Source: CAD feature listing. Evaluate the final solid. Frame: model axes, mm. A direction names the side the tool comes from. Give positions to 0.01 mm unless a question says otherwise; leave off trailing zeros. Order: outer loops, then holes, each group sorted by start corner. A loop starts at its lowest first (then second) coordinate and runs counter-clockwise, first axis right, second up. Notation, with made-up numbers: M -28.75,20 L 20.25,20 A33 ccw 20.25,49 Z; hole C 42.25,88 d8. An arc over 180 degrees is marked long. Use CSV: the item, a comma, the result in double quotes. Start each with the question number.
1. Section query B-B, the plane y = 10.5. Return the cut outline in (x, z).
2. Section query C-C, the plane x = 8.5. Return the cut outline in (y, z), plus the area to 3 significant figures.
3. Pin query (flat end, axial travel): P1, Ø0.8, axis at y = 47.5, z = 21.5, coming from the -X side; P2, Ø1.1, axis at x = 27, z = 20.5, coming from the -Y side; P3, Ø1.7, axis at x = -30, z = -17.5, coming from the -Y side; P4, Ø3, axis at y = 47.5, z = 21, coming from the +X side. Return the tip coordinate at first contact, or that it passes through.
4. Mould query, pull axis X, two halves, no side actions, for faces 4 (the flat face through (30, 2, -13)), 5 (the flat face through (-35, 29, 0)), 6 (the flat face through (0, 29, -22.5)). Classes: released by +X, released by -X, zero draft, split by the parting line, or undercut.
5. Line query: line 1 along X through (y, z) = (9, -11.5); line 2 along X through (y, z) = (1, 17); line 3 along Z through (x, y) = (-1, 14). Output: solid intervals per line, ascending. Write a range as [from, to].
6. Reachability of faces 1 (the flat face through (32.591, 30, 0)), 2 (the flat face through (-26.25, 47, 21)), 3 (the flat face through (30, 2, 13)) from +Z, -Z, +X, -X, +Y, -Y: full face, straight path, thin tool, end or side. Return the list, or none.
7. Section query D-D, the plane z = 0. Return the cut outline in (x, y).
8. Section query A-A, the plane x = 1.5. Return the cut outline in (y, z).
from build123d import *

# Parameters (mm, degrees)
SKETCH_1_W          = 70
SKETCH_1_H          = 45
EXTRUDE_1_DEPTH     = 3
SKETCH_2_W          = 13
SKETCH_2_H          = 23
CUT_EXTRUDE_1_DEPTH = 10
SKETCH_3_R          = 0.95
CUT_EXTRUDE_2_DEPTH = 10
FILLET_1_R          = 5
FILLET_2_R          = 5
SKETCH_4_R          = 0.95
CUT_EXTRUDE_3_DEPTH = 10
CUT_EXTRUDE_4_DEPTH = 10
SKETCH_9_W          = 65.182596022
SKETCH_9_H          = 39.488918008
EXTRUDE_2_DEPTH     = 55
SKETCH_10_W         = 1
SKETCH_10_H         = 2.5
SKETCH_10_W_2       = 15
SKETCH_10_H_2       = 10
CUT_EXTRUDE_5_DEPTH = 7


with BuildPart() as part:
    # 草图1 → 凸台-拉伸1 (new body)
    with BuildSketch(Plane(origin=(0, 0, 0), x_dir=(1, 0, 0), z_dir=(0, 1, 0))):
        Rectangle(SKETCH_1_W, SKETCH_1_H)
    extrude(amount=EXTRUDE_1_DEPTH)

    # 草图2 → 切除-拉伸1 (cut)
    with BuildSketch(Plane(origin=(0, 3, 0), x_dir=(1, 0, 0), z_dir=(0, 1, 0))):
        with Locations((24, 0)):
            Rectangle(SKETCH_2_W, SKETCH_2_H)
        with Locations((-24, 0)):
            Rectangle(SKETCH_2_W, SKETCH_2_H)
    extrude(amount=-CUT_EXTRUDE_1_DEPTH, mode=Mode.SUBTRACT)

    # 草图3 → 切除-拉伸2 (cut)
    with BuildSketch(Plane(origin=(0, 3, 0), x_dir=(1, 0, 0), z_dir=(0, 1, 0))):
        with Locations((-24, 14)):
            Circle(SKETCH_3_R)
        with Locations((-24, -14)):
            Circle(SKETCH_3_R)
        with Locations((24, 14)):
            Circle(SKETCH_3_R)
        with Locations((24, -14)):
            Circle(SKETCH_3_R)
    extrude(amount=-CUT_EXTRUDE_2_DEPTH, mode=Mode.SUBTRACT)

    # 圆角1
    fillet_1_edges = [part.edges().sort_by_distance(p)[0] for p in [
        (35, 1.5, -22.5),
    ]]
    fillet(fillet_1_edges, radius=FILLET_1_R)

    # 圆角2
    fillet_2_edges = [part.edges().sort_by_distance(p)[0] for p in [
        (35, 1.5, 22.5),
        (-35, 1.5, 22.5),
        (-35, 1.5, -22.5),
    ]]
    fillet(fillet_2_edges, radius=FILLET_2_R)

    # 草图4 → 切除-拉伸3 (cut)
    with BuildSketch(Plane(origin=(0, 3, 0), x_dir=(1, 0, 0), z_dir=(0, 1, 0))):
        with Locations((-30, 17.5)):
            Circle(SKETCH_4_R)
        with Locations((30, 17.5)):
            Circle(SKETCH_4_R)
        with Locations((-30, -17.5)):
            Circle(SKETCH_4_R)
        with Locations((30, -17.5)):
            Circle(SKETCH_4_R)
    extrude(amount=-CUT_EXTRUDE_3_DEPTH, mode=Mode.SUBTRACT)

    # 草图8 → 切除-拉伸4 (cut)
    with BuildSketch(Plane(origin=(0, 3, 0), x_dir=(1, 0, 0), z_dir=(0, 1, 0))):
        with BuildLine():
            Line((-27, 17.5), (27, 17.5))
            ThreePointArc((27, 17.5), (27.878679656, 15.378679656), (30, 14.5))
            Line((30, 14.5), (30, -14.5))
            ThreePointArc((30, -14.5), (27.878679656, -15.378679656), (27, -17.5))
            Line((27, -17.5), (-27, -17.5))
            ThreePointArc((-27, -17.5), (-27.878679656, -15.378679656), (-30, -14.5))
            Line((-30, -14.5), (-30, 14.5))
            ThreePointArc((-30, 14.5), (-27.878679656, 15.378679656), (-27, 17.5))
        make_face()
    extrude(amount=-CUT_EXTRUDE_4_DEPTH, mode=Mode.SUBTRACT)

    # 草图9 → 凸台-拉伸2 (add)
    with BuildSketch(Plane(origin=(0, 3, 0), x_dir=(1, 0, 0), z_dir=(0, 1, 0))):
        with BuildLine():
            Line((-30, -22.5), (30, -22.5))
            ThreePointArc((30, -22.5), (33.535533906, -21.035533906), (35, -17.5))
            Line((35, -17.5), (35, 17.5))
            ThreePointArc((35, 17.5), (33.535533906, 21.035533906), (30, 22.5))
            Line((30, 22.5), (-30, 22.5))
            ThreePointArc((-30, 22.5), (-33.535533906, 21.035533906), (-35, 17.5))
            Line((-35, 17.5), (-35, -17.5))
            ThreePointArc((-35, -17.5), (-33.535533906, -21.035533906), (-30, -22.5))
        make_face()
        Rectangle(SKETCH_9_W, SKETCH_9_H, mode=Mode.SUBTRACT)
    extrude(amount=EXTRUDE_2_DEPTH)

    # 草图10 → 切除-拉伸5 (cut)
    with BuildSketch(Plane(origin=(0, 0, 22.5), x_dir=(-1, 0, 0), z_dir=(0, 0, -1))):
        with Locations((26.75, 6.25)):
            Rectangle(SKETCH_10_W, SKETCH_10_H)
        with Locations((26.75, 47.25)):
            Rectangle(SKETCH_10_W, SKETCH_10_H)
        with Locations((-26.75, 21.25)):
            Rectangle(SKETCH_10_W, SKETCH_10_H)
        with Locations((-26.75, 47.25)):
            Rectangle(SKETCH_10_W, SKETCH_10_H)
        with Locations((0, 43)):
            Rectangle(SKETCH_10_W_2, SKETCH_10_H_2)
    extrude(amount=CUT_EXTRUDE_5_DEPTH, mode=Mode.SUBTRACT)


solid = part.part
Result set:
1,outline,"M -35,-17.5 A5 ccw -30,-22.5 L 30,-22.5 A5 ccw 35,-17.5 L 35,17.5 A5 ccw 30,22.5 L -30,22.5 A5 ccw -35,17.5 Z; hole M -32.59,-19.74 L 32.59,-19.74 L 32.59,19.74 L -32.59,19.74 Z"
2,outline,"M 0,-22.5 L 58,-22.5 L 58,-19.74 L 3,-19.74 L 3,-17.5 L 0,-17.5 Z; M 0,17.5 L 3,17.5 L 3,19.74 L 58,19.74 L 58,22.5 L 0,22.5 Z"
2,area,"333 mm2"
3,P1,"x = -33.47"
3,P2,"y = 0"
3,P3,"through"
3,P4,"x = 34.58"
4,face 4,"undercut"
4,face 5,"released by -X"
4,face 6,"zero draft"
5,line 1,"[-35, -32.59], [32.59, 35]"
5,line 2,"[-35, -30.81], [-29.19, -27.04], [27.04, 29.19], [30.81, 35]"
5,line 3,"[-22.5, -19.74], [19.74, 22.5]"
6,face 1,"+Y"
6,face 2,"+Z"
6,face 3,"+Y, -Y"
7,outline,"M -35,0 L -30.5,0 L -30.5,3 L -32.59,3 L -32.59,58 L -35,58 Z; M 30.5,0 L 35,0 L 35,58 L 32.59,58 L 32.59,3 L 30.5,3 Z"
8,outline,"M 0,-22.5 L 58,-22.5 L 58,-19.74 L 3,-19.74 L 3,-17.5 L 0,-17.5 Z; M 0,17.5 L 3,17.5 L 3,19.74 L 38,19.74 L 38,22.5 L 0,22.5 Z; M 48,19.74 L 58,19.74 L 58,22.5 L 48,22.5 Z"
